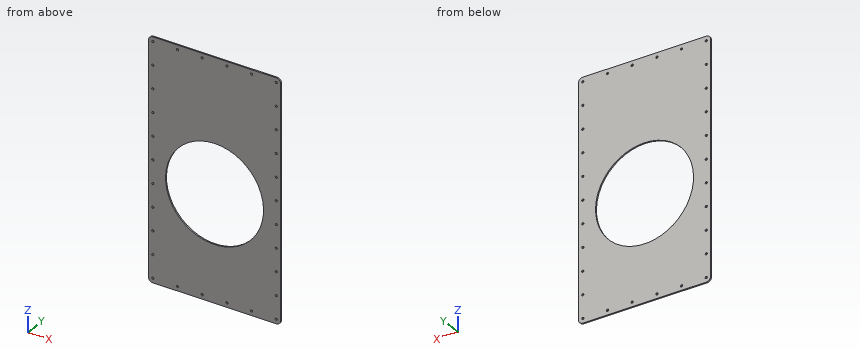
```python
from build123d import *

# Parameters (mm, degrees)
SKETCH9_W               = 300
SKETCH9_H               = 540
SKETCH9_R               = 2.5
BOSS_EXTRUDE7_DEPTH     = 3.175
FILLET4_R               = 10
CUT_EXTRUDE1_DEPTH      = 543.618724912
CUT_EXTRUDE1_DEPTH_BACK = 543.618724912
SKETCH9_3_R             = 111.125


with BuildPart() as part:
    # Sketch9 → Boss-Extrude7 (new body)
    with BuildSketch(Plane(origin=(0, 0, 0), x_dir=(1, 0, 0), z_dir=(0, 1, 0))):
        with Locations((5, 250)):
            Rectangle(SKETCH9_W, SKETCH9_H)
        with Locations(Location((-135, -10, 0), (0, 0, 270))):
            Circle(SKETCH9_R, mode=Mode.SUBTRACT)
        with Locations(Location((-135, 42, 0), (0, 0, 270))):
            Circle(SKETCH9_R, mode=Mode.SUBTRACT)
        with Locations(Location((-135, 94, 0), (0, 0, 270))):
            Circle(SKETCH9_R, mode=Mode.SUBTRACT)
        with Locations(Location((-135, 146, 0), (0, 0, 270))):
            Circle(SKETCH9_R, mode=Mode.SUBTRACT)
        with Locations(Location((-135, 198, 0), (0, 0, 270))):
            Circle(SKETCH9_R, mode=Mode.SUBTRACT)
        with Locations(Location((-135, 250, 0), (0, 0, 270))):
            Circle(SKETCH9_R, mode=Mode.SUBTRACT)
        with Locations(Location((-135, 302, 0), (0, 0, 270))):
            Circle(SKETCH9_R, mode=Mode.SUBTRACT)
        with Locations(Location((-135, 354, 0), (0, 0, 270))):
            Circle(SKETCH9_R, mode=Mode.SUBTRACT)
        with Locations(Location((-135, 406, 0), (0, 0, 270))):
            Circle(SKETCH9_R, mode=Mode.SUBTRACT)
        with Locations(Location((-135, 458, 0), (0, 0, 270))):
            Circle(SKETCH9_R, mode=Mode.SUBTRACT)
        with Locations(Location((-135, 510, 0), (0, 0, 270))):
            Circle(SKETCH9_R, mode=Mode.SUBTRACT)
        with Locations(Location((-79, 510, 0), (0, 0, 270))):
            Circle(SKETCH9_R, mode=Mode.SUBTRACT)
        with Locations(Location((-23, 510, 0), (0, 0, 270))):
            Circle(SKETCH9_R, mode=Mode.SUBTRACT)
        with Locations(Location((33, 510, 0), (0, 0, 270))):
            Circle(SKETCH9_R, mode=Mode.SUBTRACT)
        with Locations(Location((89, 510, 0), (0, 0, 270))):
            Circle(SKETCH9_R, mode=Mode.SUBTRACT)
        with Locations(Location((145, 510, 0), (0, 0, 270))):
            Circle(SKETCH9_R, mode=Mode.SUBTRACT)
        with Locations(Location((145, 458, 0), (0, 0, 270))):
            Circle(SKETCH9_R, mode=Mode.SUBTRACT)
        with Locations(Location((145, 406, 0), (0, 0, 270))):
            Circle(SKETCH9_R, mode=Mode.SUBTRACT)
        with Locations(Location((145, 354, 0), (0, 0, 270))):
            Circle(SKETCH9_R, mode=Mode.SUBTRACT)
        with Locations(Location((145, 302, 0), (0, 0, 270))):
            Circle(SKETCH9_R, mode=Mode.SUBTRACT)
        with Locations(Location((145, 250, 0), (0, 0, 270))):
            Circle(SKETCH9_R, mode=Mode.SUBTRACT)
        with Locations(Location((145, 198, 0), (0, 0, 270))):
            Circle(SKETCH9_R, mode=Mode.SUBTRACT)
        with Locations(Location((145, 146, 0), (0, 0, 270))):
            Circle(SKETCH9_R, mode=Mode.SUBTRACT)
        with Locations(Location((145, 94, 0), (0, 0, 270))):
            Circle(SKETCH9_R, mode=Mode.SUBTRACT)
        with Locations(Location((145, 42, 0), (0, 0, 270))):
            Circle(SKETCH9_R, mode=Mode.SUBTRACT)
        with Locations(Location((145, -10, 0), (0, 0, 270))):
            Circle(SKETCH9_R, mode=Mode.SUBTRACT)
        with Locations(Location((89, -10, 0), (0, 0, 270))):
            Circle(SKETCH9_R, mode=Mode.SUBTRACT)
        with Locations(Location((33, -10, 0), (0, 0, 270))):
            Circle(SKETCH9_R, mode=Mode.SUBTRACT)
        with Locations(Location((-23, -10, 0), (0, 0, 270))):
            Circle(SKETCH9_R, mode=Mode.SUBTRACT)
        with Locations(Location((-79, -10, 0), (0, 0, 270))):
            Circle(SKETCH9_R, mode=Mode.SUBTRACT)
    extrude(amount=BOSS_EXTRUDE7_DEPTH)

    # Fillet4
    fillet4_edges = [part.edges().sort_by_distance(p)[0] for p in [
        (155, 1.5875, -520),
        (155, 1.5875, 20),
        (-145, 1.5875, 20),
        (-145, 1.5875, -520),
    ]]
    fillet(fillet4_edges, radius=FILLET4_R)

    # Sketch9_3 → Cut-Extrude1 (cut, two sides: drawn at the far end of the back side and taken through both)
    with BuildSketch(Plane(origin=(0, 0, 0), x_dir=(1, 0, 0), z_dir=(0, 1, 0)).offset(-CUT_EXTRUDE1_DEPTH_BACK)):
        with Locations(Location((5, 280, 0), (0, 0, 270))):
            Circle(SKETCH9_3_R)
    extrude(amount=CUT_EXTRUDE1_DEPTH + CUT_EXTRUDE1_DEPTH_BACK, mode=Mode.SUBTRACT)


solid = part.part
```
Design review of the part built by this model. Coordinates are the model's own, in mm. Coordinates: 2 decimals unless noted, no trailing zeros. Loops run counter-clockwise (first coordinate to the right, second up) from the corner with the lowest first, then second, coordinate; pieces in that order, holes last. Notation, with made-up numbers: (2.5, 24.25) - (19.5, 24.25) arc R13 ccw to (19.5, 33.25) - close; hole circle Ø9 at (72.5, -9). An arc over 180 degrees is marked (long way). Use CSV: the item, a comma, the result in double quotes. Start each with the question number.
1) Consider section C-C on y = 0.95. Give the number of separate pieces and of enclosed holes in the cut face, then the cut area to 3 significant figures.
2) Consider section A-A on x = 5. Write out the cut boundary in (y, z) (3 decimals).
3) Consider section B-B on z = -293. Write out the cut boundary in (x, y) (3 decimals), then the cut area to 3 significant figures.
4) Wall thickness on L1, parallel to X at y = 1.45, z = -406; L2, parallel to X at y = 2, z = -302; L3, parallel to X at y = 1.4, z = -93: over which ranges is each line inside the solid? List them lowest first. Write a range as from..to.
Geometry says:
1,separate pieces,"1"
1,enclosed holes,"31"
1,area,"123,000 mm^2"
2,outline,"(0, -520) - (3.175, -520) - (3.175, -391.125) - (0, -391.125) - close; (0, -168.875) - (3.175, -168.875) - (3.175, 20) - (0, 20) - close"
3,outline,"(-145, 0) - (-105.362, 0) - (-105.362, 3.175) - (-145, 3.175) - close; (115.362, 0) - (155, 0) - (155, 3.175) - (115.362, 3.175) - close"
3,area,"252 mm^2"
4,L1,"-145..-137.5, -132.5..142.5, 147.5..155"
4,L2,"-145..-137.5, -132.5..-103.93, 113.93..142.5, 147.5..155"
4,L3,"-145..-137.29, -132.71..142.71, 147.29..155"
